```python
from build123d import *

# Parameters (mm, degrees)
F1_DEPTH  = 25.4
F2_W      = 57.15
F2_H      = 31.75
F3_DEPTH  = 57.15
F4_W      = 6.35
F4_H      = 6.35
F5_DEPTH  = 57.151
F4_W_2    = 12.7
F4_H_2    = 12.7
F6_DEPTH  = 31.75
F6_FACE_W = 12.7
F6_FACE_H = 12.7
F7_DEPTH  = 25.401
F8_R      = 6.35
F9_DEPTH  = 25.401
F10_SIZE  = 17.78


with BuildPart() as f1:
    # F0 (on Front) → F1 (new body)
    with BuildSketch(Plane.XZ):
        Polygon((0, 50.8), (0, 0), (107.95, 0), (107.95, 19.05), (50.8, 50.8), align=None)
    extrude(amount=F1_DEPTH)

    # F2 (on Front) → F3 (join)
    with BuildSketch(Plane.XZ):
        with Locations((28.575, 3.175)):
            Rectangle(F2_W, F2_H)
    extrude(amount=F3_DEPTH)

    # F4 (on face) → F5 (cut, through all)
    with BuildSketch(Plane.XZ.offset(57.15)):
        with Locations((3.175, -9.525)):
            Rectangle(F4_W, F4_H)
    extrude(amount=-F5_DEPTH, mode=Mode.SUBTRACT)

    # F4 (on face) → F6 (cut)
    with BuildSketch(Plane.XZ.offset(57.15)):
        with Locations((50.8, 12.7)):
            Rectangle(F4_W_2, F4_H_2)
        with Locations((50.8, -6.35)):
            Rectangle(F4_W_2, F4_H_2)
    extrude(amount=-F6_DEPTH, mode=Mode.SUBTRACT)

    # F6_face (on face) → F7 (cut, through all)
    with BuildSketch(Plane(origin=(50.8, -25.4, -6.35), x_dir=(1, 0, 0), z_dir=(0, -1, 0))):
        Rectangle(F6_FACE_W, F6_FACE_H)
    extrude(amount=-F7_DEPTH, mode=Mode.SUBTRACT)

    # F8 (on face) → F9 (cut, through all)
    with BuildSketch(Plane.XZ.offset(25.4)):
        with Locations((19.05, 38.1)):
            Circle(F8_R)
    extrude(amount=-F9_DEPTH, mode=Mode.SUBTRACT)

    # F10
    f10_edges = [f1.edges().sort_by_distance(p)[0] for p in [
        (107.95, 0, 9.525),
    ]]
    chamfer(f10_edges, length=F10_SIZE)


solid = f1.part
```
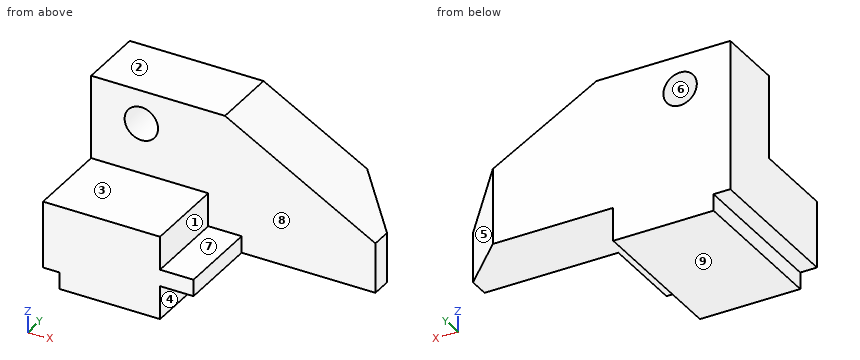
Model file for the job. Use its own axes, mm. Face numbers are marked on the shaded views. A direction names the side the tool comes from. Give positions to 0.01 mm unless a question says otherwise; leave off trailing zeros. Loops run counter-clockwise (first coordinate to the right, second up) from the corner with the lowest first, then second, coordinate; pieces in that order, holes last. Notation, with made-up numbers: M 4.5,31 L 36.5,31 A15 cw 36.5,53 Z; hole C 59,84 d3. An arc over 180 degrees is marked long. Use one line per item in the form item = value.
Item 1: Flat gauge pins, fed straight in: pin 1 Ø4 at (y, z) = (-33.5, -5.5) entering from +X; pin 2 Ø14 at (x, y) = (48, -33.5) entering from +Z; pin 3 Ø7.5 at (x, z) = (19.05, 38.1) entering from +Y; pin 4 Ø2 at (y, z) = (-43, 1.5) entering from -X. Where does each tip first touch, or does it go through?
Filled in:
pin_1 = 44.45
pin_2 = 19.05
pin_3 = through
pin_4 = 0
Item 2: Slice it at B-B on x = 19.05. List the corners of the cut face in (y, z).
Filled in:
outline = M -57.15,-12.7 L 0,-12.7 L 0,31.75 L -25.4,31.75 L -25.4,19.05 L -57.15,19.05 Z; M -25.4,44.45 L 0,44.45 L 0,50.8 L -25.4,50.8 Z
Item 3: Which spindle directions (+Z, -Z, +X, -X, +Y, -Y) get a long thin tool onto all of the face, cutting with end or side? Do the marked faces 1, 2, 3, 4 and 5. Say none if no direction does.
Filled in:
face_1 = +Z, +X, -Y
face_2 = +Z, +X, -X, +Y, -Y
face_3 = +Z, +X, -X, -Y
face_4 = -Z, +X, +Y, -Y
face_5 = +Z, -Z, +X, +Y
Item 4: Slice it at A-A on z = 38.1. List the corners of the cut face in (x, y), and give its area (3 significant figures).
Filled in:
outline = M 0,-25.4 L 12.7,-25.4 L 12.7,0 L 0,0 Z; M 25.4,-25.4 L 73.66,-25.4 L 73.66,0 L 25.4,0 Z
area = 1,550 mm^2
Item 5: Slice it at D-D on y = -37.5. List the corners of the cut face in (x, z), and give its area (3 significant figures).
Filled in:
outline = M 0,-6.35 L 6.35,-6.35 L 6.35,-12.7 L 44.45,-12.7 L 44.45,0 L 57.15,0 L 57.15,6.35 L 44.45,6.35 L 44.45,19.05 L 0,19.05 Z
area = 1,450 mm^2
Item 6: Slice it at C-C on y = -5. List the corners of the cut face in (x, z).
Filled in:
outline = M 0,-6.35 L 6.35,-6.35 L 6.35,-12.7 L 44.45,-12.7 L 44.45,0 L 95.17,0 L 95.17,26.15 L 50.8,50.8 L 0,50.8 Z; hole C 19.05,38.1 d12.7
Item 7: Drill centre lines: L1, parallel to Z at x = 19.05, y = -9.5; L2, parallel to X at y = -29, z = 2.5; L3, parallel to Z at x = 34, y = -34.5. Where is each one in solid material? Low to high.
Filled in:
L1 = -12.7 to 31.75, 44.45 to 50.8
L2 = 0 to 57.15
L3 = -12.7 to 19.05
Item 8: Two-plate mould, pull along Z, no slides. Class the marked faces 6, 7, 8 and 9: released by +Z, released by -Z, zero draft, split by the parting line, or undercut.
Filled in:
face_6 = undercut
face_7 = released by +Z
face_8 = zero draft
face_9 = released by -Z
